from build123d import *

# Parameters (mm, degrees)
SKETCH1_W           = 178
SKETCH1_H           = 80
BOSS_EXTRUDE1_DEPTH = 6.6
FILLET1_R           = 5
SKETCH5_W           = 32
SKETCH5_H           = 7.6
CUT_EXTRUDE1_DEPTH  = 6.6
SKETCH13_R          = 2
BOSS_EXTRUDE2_DEPTH = 4
BOSS_EXTRUDE2_TAPER = 15
SKETCH10_R          = 2
BOSS_EXTRUDE5_DEPTH = 4
BOSS_EXTRUDE5_TAPER = 15
SKETCH9_R           = 2
BOSS_EXTRUDE6_DEPTH = 4
BOSS_EXTRUDE6_TAPER = 15
SKETCH6_R           = 2
BOSS_EXTRUDE9_DEPTH = 3
BOSS_EXTRUDE9_TAPER = 15
ZAOBLIT4_R          = 2


with BuildPart() as part:
    # Sketch1 → Boss-Extrude1 (new body)
    with BuildSketch(Plane.XY):
        with Locations((89, 40)):
            Rectangle(SKETCH1_W, SKETCH1_H)
    extrude(amount=BOSS_EXTRUDE1_DEPTH)

    # Fillet1
    fillet1_edges = [part.edges().sort_by_distance(p)[0] for p in [
        (0, 80, 3.3),
        (178, 80, 3.3),
        (178, 0, 3.3),
        (0, 0, 3.3),
    ]]
    fillet(fillet1_edges, radius=FILLET1_R)

    # Sketch5 → Cut-Extrude1 (cut)
    with BuildSketch(Plane.XY.offset(6.6)):
        with Locations((23, 76.2)):
            Rectangle(SKETCH5_W, SKETCH5_H)
        with Locations((155, 76.2)):
            Rectangle(SKETCH5_W, SKETCH5_H)
    extrude(amount=-CUT_EXTRUDE1_DEPTH, mode=Mode.SUBTRACT)

    # Sketch13 → Boss-Extrude2 (add)
    with BuildSketch(Plane(origin=(139, 0, 0), x_dir=(0, 0, -1), z_dir=(1, 0, 0))):
        with Locations((-3.3, 76.7)):
            Circle(SKETCH13_R)
    extrude(amount=BOSS_EXTRUDE2_DEPTH, taper=BOSS_EXTRUDE2_TAPER)

    # Sketch10 → Boss-Extrude5 (add)
    with BuildSketch(Plane(origin=(7, 0, 0), x_dir=(0, 0, -1), z_dir=(1, 0, 0))):
        with Locations((-3.3, 76.7)):
            Circle(SKETCH10_R)
    extrude(amount=BOSS_EXTRUDE5_DEPTH, taper=BOSS_EXTRUDE5_TAPER)

    # Sketch9 → Boss-Extrude6 (add)
    with BuildSketch(Plane.ZY.offset(-39)):
        with Locations((3.3, 76.7)):
            Circle(SKETCH9_R)
    extrude(amount=BOSS_EXTRUDE6_DEPTH, taper=BOSS_EXTRUDE6_TAPER)

    # Sketch6 → Boss-Extrude9 (add)
    with BuildSketch(Plane.ZY.offset(-171)):
        with Locations((3.3, 76.7)):
            Circle(SKETCH6_R)
    extrude(amount=BOSS_EXTRUDE9_DEPTH, taper=BOSS_EXTRUDE9_TAPER)

    # Zaoblit4
    zaoblit4_edges = [part.edges().sort_by_distance(p)[0] for p in [
        (172, 80, 0),
        (172, 80, 6.6),
        (0, 40, 0),
        (178, 40, 0),
        (89, 0, 0),
        (1.464466094, 1.464466094, 0),
        (176.535533906, 1.464466094, 0),
        (1.464466094, 78.535533906, 0),
        (176.535533906, 78.535533906, 0),
        (178, 40, 6.6),
        (0, 40, 6.6),
        (89, 0, 6.6),
        (1.464466094, 1.464466094, 6.6),
        (176.535533906, 1.464466094, 6.6),
        (1.464466094, 78.535533906, 6.6),
        (176.535533906, 78.535533906, 6.6),
        (89, 80, 0),
        (6, 80, 0),
        (89, 80, 6.6),
        (6, 80, 6.6),
    ]]
    fillet(zaoblit4_edges, radius=ZAOBLIT4_R)


solid = part.part
CAD build for the part. Positions are in the model's coordinates, mm. A direction names the side the tool comes from. Coordinates: 2 decimals unless noted, no trailing zeros. Loops run counter-clockwise (first coordinate to the right, second up) from the corner with the lowest first, then second, coordinate; pieces in that order, holes last. Notation, with made-up numbers: (83.5, 86.5) - (109.5, 86.5) arc R16 ccw to (109.5, 112.5) - close; hole circle Ø5 at (28, 66.5). An arc over 180 degrees is marked (long way). Write item = value, one per line. Start each with the question number.
Q1. Which spindle directions (+Z, -Z, +X, -X, +Y, -Y) get a long thin tool onto all of the face, cutting with end or side? Do faces 1 (the cylindrical face through (177, 78, 3)), 2 (the flat face through (171, 74, 3)). Say none if no direction does.
Q2. Cut at A-A, the plane x = 32. List the corners of the cut face in (y, z).
Q3. Flat gauge pins, fed straight in: pin 1 Ø2 at (y, z) = (76.5, 3) entering from -X; pin 2 Ø3.5 at (x, z) = (154.5, 2.5) entering from +Y; pin 3 Ø2 at (y, z) = (77, 3.5) entering from +X. Where does each tip first touch, or does it go through?
Q4. Drill centre lines: L1, parallel to X at y = 54, z = 1.75; L2, parallel to Y at x = 19, z = 1.25; L3, parallel to X at y = 61, z = 0.75. Where is each one in solid material? Low to high.
Q5. Pull direction Y, two halves, no side cores. Call faces 3 (the cylindrical face through (1, 78, 3)), 4 (the cylindrical face through (176, 1, 3)), 5 (the conical face through (141.472, 78.026, 3.474)): pulls with the +Y half, pulls with the -Y half, needs draft (parallel to the pull), parting line crosses it, or undercut.
Computed:
q1.face_1 = +Z, -Z, +X, +Y
q1.face_2 = none
q2.outline = (0, 2) arc R2 ccw to (2, 0) - (72.4, 0) - (72.4, 6.6) - (2, 6.6) arc R2 ccw to (0, 4.6) - close
q3.pin_1 = 0.03
q3.pin_2 = 72.4
q3.pin_3 = 177.9
q4.L1 = 0.02 to 177.98
q4.L2 = 0.15 to 72.4
q4.L3 = 0.44 to 177.56
q5.face_3 = pulls with the +Y half
q5.face_4 = pulls with the -Y half
q5.face_5 = undercut
